Check sheet for the modelled part. Datum: model origin and axes. Units: mm. A direction names the side the tool comes from. Round coordinates to 2 decimals unless told otherwise and drop trailing zeros. Loops run counter-clockwise (first coordinate to the right, second up) from the corner with the lowest first, then second, coordinate; pieces in that order, holes last. Notation, with made-up numbers: (50.25, -15) -> (79.25, -15) arc R19 cw to (79.25, 14) -> close; hole circle Ø7 at (9.25, -10). An arc over 180 degrees is marked (long way). Use one line per item in the form item = value. Start each with the question number.
(1) Material ranges on probe 1 along X at (y, z) = (6.25, 0.3); probe 2 along X at (y, z) = (11.5, 1.8); probe 3 along X at (y, z) = (2.75, 1.45), recorded low to high. Write a range as [from, to].
(2) Draft check along X on faces 1 (the flat face through (5, 16, 1)), 2 (the flat face through (29.43, 15.63, 0.99)), 3 (the flat face through (19.022, 2, 1)), 4 (the flat face through (22, 7, 2)). Enter one of: released by +X, released by -X, zero draft, split by the parting line, or undercut.
(3) Sectioned sample at D-D (x = 25). Record the cut outline in (y, z), and give its area (3 significant figures).
(4) Sectioned sample at C-C (x = 35). Record the cut outline in (y, z), and give its area (3 significant figures).
(5) Go/stop test with flat-tipped pins: pin 1 (1 mm diameter, centred on y = 15.5, z = 0.5, fed in from -X); pin 2 (1.8 mm diameter, centred on x = 3.92, y = 9, fed in from +Z); pin 3 (1 mm diameter, centred on x = 10, z = 0.5, fed in from -Y); pin 4 (1 mm diameter, centred on x = 23, z = 1.5, fed in from +Y). Record where each tip stops, or that it passes through.
(6) Sectioned sample at B-B (z = 1.15). State how many separate pieces and enclosed holes the cut face has, and give its area (3 significant figures).
(7) Set-up check for faces 5 (the flat face through (3, 14, 1)), 6 (the flat face through (16.643, 5.714, 0.986)), 7 (the flat face through (18, 4, 1)): record each of +Z, -Z, +X, -X, +Y, -Y from which the full face is reachable in a straight line by a thin tool's end or side.
(8) Sectioned sample at A-A (y = 9). Record the cut outline in (x, z), and give its area (3 significant figures).
from build123d import *

# Parameters (mm, degrees)
SKETCH1_R           = 1.5
BOSS_EXTRUDE1_DEPTH = 2


with BuildPart() as part:
    # Sketch1 → Boss-Extrude1 (new body)
    with BuildSketch(Plane.XY):
        with BuildLine():
            Line((5, 0), (9, 0))
            Line((9, 0), (9, 4))
            Line((9, 4), (13, 4))
            Line((13, 4), (13, 0))
            Line((13, 0), (17, 0))
            Line((17, 0), (17, 4))
            Line((17, 4), (19.021561934, 4))
            Line((19.021561934, 4), (19.021561934, 0))
            Line((19.021561934, 0), (38.059495851, 0))
            ThreePointArc((38.059495851, 0), (44.762590659, 5.991570372), (39.557599026, 13.322222296))
            Line((39.557599026, 13.322222296), (19.021561934, 17.999988357))
            Line((19.021561934, 17.999988357), (19.021561934, 13.999988357))
            Line((19.021561934, 13.999988357), (17, 13.999988357))
            Line((17, 13.999988357), (17, 17.999988357))
            Line((17, 17.999988357), (13, 17.999988357))
            Line((13, 17.999988357), (13, 13.999988357))
            Line((13, 13.999988357), (9, 13.999988357))
            Line((9, 13.999988357), (9, 17.999988357))
            Line((9, 17.999988357), (5, 17.999988357))
            Line((5, 17.999988357), (5, 13.999988357))
            Line((5, 13.999988357), (0, 13.999988357))
            Line((0, 13.999988357), (0, 4))
            Line((0, 4), (5, 4))
            Line((5, 4), (5, 0))
        make_face()
        with Locations((3.920490093, 9)):
            Circle(SKETCH1_R, mode=Mode.SUBTRACT)
        with Locations((38.059495851, 6.745343083)):
            Circle(SKETCH1_R, mode=Mode.SUBTRACT)
        Polygon((23.639149333, 12.024852982), (21.669533827, 11.677556626), (22.537774715, 6.753517861), (24.507390221, 7.100814216), align=None, mode=Mode.SUBTRACT)
        Polygon((16.745495062, 10.809315738), (17.61373595, 5.885276973), (15.644120444, 5.537980617), (14.775879556, 10.462019383), align=None, mode=Mode.SUBTRACT)
    extrude(amount=BOSS_EXTRUDE1_DEPTH)


solid = part.part
Checks:
q1.probe_1 = [0, 15.52], [17.55, 36.64], [39.48, 44.79]
q1.probe_2 = [0, 21.7], [23.73, 42.84]
q1.probe_3 = [5, 9], [13, 17], [19.02, 43.49]
q2.face_1 = released by -X
q2.face_2 = released by +X
q2.face_3 = undercut
q2.face_4 = zero draft
q3.outline = (0, 0) -> (16.64, 0) -> (16.64, 2) -> (0, 2) -> close
q3.area = 33.3 mm2
q4.outline = (0, 0) -> (14.36, 0) -> (14.36, 2) -> (0, 2) -> close
q4.area = 28.7 mm2
q5.pin_1 = 5
q5.pin_2 = through
q5.pin_3 = 4
q5.pin_4 = 17.21
q6.separate_pieces = 1
q6.enclosed_holes = 4
q6.area = 593 mm2
q7.face_5 = +Z, -Z, -X, +Y
q7.face_6 = +Z, -Z
q7.face_7 = +Z, -Z, -Y
q8.outline = (0, 0) -> (2.42, 0) -> (2.42, 2) -> (0, 2) -> close; (5.42, 0) -> (15.03, 0) -> (15.03, 2) -> (5.42, 2) -> close; (17.06, 0) -> (22.14, 0) -> (22.14, 2) -> (17.06, 2) -> close; (24.17, 0) -> (44.42, 0) -> (44.42, 2) -> (24.17, 2) -> close
q8.area = 74.7 mm2
